Source: three-view drawing plus pictorial views. Frame: mm from the lowest corner of the part. A direction names the side the tool comes from. Give positions to 0.01 mm unless a question says otherwise; leave off trailing zeros. Order: outer loops, then holes, each group sorted by start corner. A loop starts at its lowest first (then second) coordinate and runs counter-clockwise, first axis right, second up.
1) Section A-A, the plane z = 46. Return loops of the section in (x, y).
2) Section B-B, the plane x = 5.5. Return loops of the section in (y, z).
3) Access query for the marked faces 1, 2 and 3. Directions: +Z, -Z, +X, -X, +Y, -Y. A direction counts if a zero-diameter tool reaches every point of the face in a straight line with its end or side. Return the directions, or none.
4) Draft query along Z for the marked faces 4, 5 and 6. Return one class per face: released by +Z, released by -Z, zero draft, split by the parting line, or undercut.
5) First-contact query: P1, Ø1.6, axis at y = 22, z = 1, coming from the -X side; P2, Ø12, axis at x = 6, y = 8.5, coming from the -Z side; P3, Ø2, axis at y = 28, z = 0.5, coming from the +X side. Flat tips, straight axial feed; report the tip coordinate or a pass-through.
6) Section C-C, the plane y = 6.5. Return loops of the section in (x, z), plus the area to 3 significant figures.
7) Material intervals for line 1 (X direction, y = 11.5, z = 61); line 2 (Z direction, x = 14, y = 7.5); line 3 (Z direction, x = 36.5, y = 10), sorted ascending.
8) Section D-D, the plane x = 23.5. Return loops of the section in (y, z).
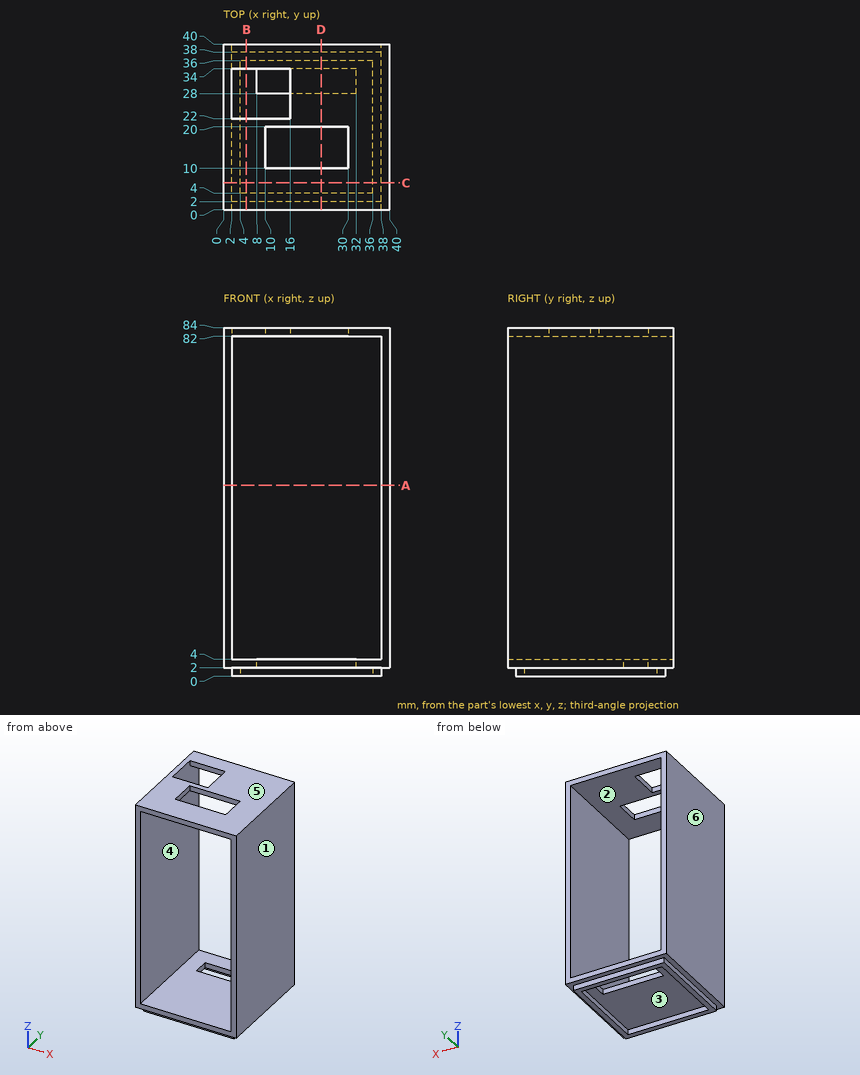
From the geometry:
1. outline: (0, 0) - (2, 0) - (2, 40) - (0, 40) - close; (38, 0) - (40, 0) - (40, 40) - (38, 40) - close
2. outline: (0, 2) - (2, 2) - (2, 0) - (4, 0) - (4, 2) - (36, 2) - (36, 0) - (38, 0) - (38, 2) - (40, 2) - (40, 4) - (0, 4) - close; (0, 82) - (22, 82) - (22, 84) - (0, 84) - close; (34, 82) - (40, 82) - (40, 84) - (34, 84) - close
3. face 1: +Z, -Z, +X, +Y, -Y
3. face 2: +Y, -Y
3. face 3: -Z
4. face 4: undercut
4. face 5: released by +Z
4. face 6: zero draft
5. P1: stops at x = 2
5. P2: stops at z = 0
5. P3: stops at x = 38
6. outline: (0, 2) - (2, 2) - (2, 0) - (4, 0) - (4, 2) - (36, 2) - (36, 0) - (38, 0) - (38, 2) - (40, 2) - (40, 84) - (0, 84) - close; hole (2, 4) - (38, 4) - (38, 82) - (2, 82) - close
6. area: 480 mm2
7. line 1: x = 0 to 2, 38 to 40
7. line 2: z = 2 to 4, 82 to 84
7. line 3: z = 0 to 4, 82 to 84
8. outline: (0, 2) - (2, 2) - (2, 0) - (4, 0) - (4, 2) - (28, 2) - (28, 4) - (0, 4) - close; (0, 82) - (10, 82) - (10, 84) - (0, 84) - close; (20, 82) - (40, 82) - (40, 84) - (20, 84) - close; (34, 2) - (36, 2) - (36, 0) - (38, 0) - (38, 2) - (40, 2) - (40, 4) - (34, 4) - close
